CAD build for the part. Positions are in the model's coordinates, mm. A direction names the side the tool comes from. Give positions to 0.01 mm unless a question says otherwise; leave off trailing zeros. Write each loop counter-clockwise with the first axis right and the second up, starting at its lowest first coordinate (ties: lowest second). Pieces come first, ordered by that corner, then holes. Notation, with made-up numbers: (43, 55.5) - (86, 55.5) arc R11 ccw to (86, 69.5) - close; hole circle Ø5 at (23, -24). An arc over 180 degrees is marked (long way). Put each result on its own line as item: value. Start each with the question number.
1. Cut at A-A on y = -3.75. List the corners of the cut face in (x, z).
2. Cut at B-B on y = 6.5. List the corners of the cut face in (x, z), and give its area (3 significant figures).
3. Mould opens along Y. For faces 6 (the cylindrical face through (-7.166, -0.243, 4.93)), 7 (the cylindrical face through (5.31, -4.78, 4.93)), 8 (the cylindrical face through (-0.947, 8.846, 4.93)) say: +Y half, -Y half, draft (parallel to the pull), parting line (faces both ways), or undercut.
4. Drop flat-ended pins along their axis: pin 1 (1.5 mm diameter, centred on y = 3, z = 5, fed in from +X); pin 2 (5 mm diameter, centred on x = -7, z = 4.5, fed in from +Y); pin 3 (2 mm diameter, centred on x = -1.5, y = -1.5, fed in from -Z). Give the stop position or say it passes through.
5. Wall check: line 1 (X direction, y = 6.5, z = 7.25); line 2 (X direction, y = 5.75, z = 6); line 3 (X direction, y = -7.5, z = 7.5). Give the ranges that are in metal, low to high.
6. Tool access for faces 1 (the cylindrical face through (5.37, 2.46, 4.93)), 2 (the cylindrical face through (-2.14, -8.64, 4.93)), 3 (the cylindrical face through (-3.36, 6.31, 4.93)), 4 (the cylindrical face through (-3.8, -6.1, 4.9)), 5 (the cylindrical face through (8.85, 0.58, 4.93)): list every direction of +Z, -Z, +X, -X, +Y, -Y with a clear straight run to the whole face (end or side of a thin tool).
from build123d import *

# Parameters (mm, degrees)
F1_DEPTH = 10


with BuildPart() as f1:
    # F0 (on Top) → F1 (new body)
    with BuildSketch(Plane.XY):
        with BuildLine():
            ThreePointArc((1.864316, 5.3522), (1.490455, 5.713083), (1.417156, 6.227511))
            ThreePointArc((1.417156, 6.227511), (1.483836, 7.003606), (1.389552, 7.776834))
            ThreePointArc((1.389552, 7.776834), (0.955753, 8.832789), (0.188574, 9.678163))
            Line((0.188574, 9.678163), (0, 9.68))
            Line((0, 9.68), (-0.188574, 9.678163))
            ThreePointArc((-0.188574, 9.678163), (-0.955753, 8.832789), (-1.389552, 7.776834))
            ThreePointArc((-1.389552, 7.776834), (-1.483836, 7.003606), (-1.417156, 6.227511))
            ThreePointArc((-1.417156, 6.227511), (-1.490455, 5.713083), (-1.864316, 5.3522))
            ThreePointArc((-1.864316, 5.3522), (-1.900395, 5.336418), (-1.937206, 5.32243))
            ThreePointArc((-1.937206, 5.32243), (-1.974396, 5.309483), (-2.012179, 5.298382))
            ThreePointArc((-2.012179, 5.298382), (-2.530544, 5.334521), (-2.917363, 5.68148))
            ThreePointArc((-2.917363, 5.68148), (-3.365147, 6.318865), (-3.934394, 6.850587))
            ThreePointArc((-3.934394, 6.850587), (-4.945458, 7.380655), (-6.076547, 7.535116))
            Line((-6.076547, 7.535116), (-6.222184, 7.41531))
            Line((-6.222184, 7.41531), (-6.365459, 7.29269))
            ThreePointArc((-6.365459, 7.29269), (-6.409757, 6.151962), (-6.063311, 5.064213))
            ThreePointArc((-6.063311, 5.064213), (-5.638516, 4.411282), (-5.088571, 3.85962))
            ThreePointArc((-5.088571, 3.85962), (-4.814053, 3.418429), (-4.868477, 2.901664))
            ThreePointArc((-4.868477, 2.901664), (-4.88597, 2.866383), (-4.905178, 2.832006))
            ThreePointArc((-4.905178, 2.832006), (-4.925345, 2.798183), (-4.947153, 2.765393))
            ThreePointArc((-4.947153, 2.765393), (-5.367473, 2.459878), (-5.886814, 2.477022))
            ThreePointArc((-5.886814, 2.477022), (-6.63954, 2.677457), (-7.417393, 2.718875))
            ThreePointArc((-7.417393, 2.718875), (-8.532634, 2.475031), (-9.498384, 1.866304))
            Line((-9.498384, 1.866304), (-9.532939, 1.680914))
            Line((-9.532939, 1.680914), (-9.563876, 1.494886))
            ThreePointArc((-9.563876, 1.494886), (-8.864564, 0.592564), (-7.899979, -0.018009))
            ThreePointArc((-7.899979, -0.018009), (-7.154871, -0.24513), (-6.378987, -0.31423))
            ThreePointArc((-6.378987, -0.31423), (-5.885103, -0.475745), (-5.594623, -0.906593))
            ThreePointArc((-5.594623, -0.906593), (-5.585346, -0.944864), (-5.577963, -0.983545))
            ThreePointArc((-5.577963, -0.983545), (-5.571671, -1.022419), (-5.567299, -1.061555))
            ThreePointArc((-5.567299, -1.061555), (-5.692902, -1.56577), (-6.10176, -1.886463))
            ThreePointArc((-6.10176, -1.886463), (-6.807219, -2.216763), (-7.429712, -2.685029))
            ThreePointArc((-7.429712, -2.685029), (-8.127296, -3.588688), (-8.475822, -4.675772))
            Line((-8.475822, -4.675772), (-8.383126, -4.84))
            Line((-8.383126, -4.84), (-8.287248, -5.002391))
            ThreePointArc((-8.287248, -5.002391), (-7.171543, -5.244101), (-6.04016, -5.091804))
            ThreePointArc((-6.04016, -5.091804), (-5.323383, -4.786843), (-4.684605, -4.341048))
            ThreePointArc((-4.684605, -4.341048), (-4.202447, -4.147313), (-3.702983, -4.290645))
            ThreePointArc((-3.702983, -4.290645), (-3.671276, -4.313999), (-3.640757, -4.338885))
            ThreePointArc((-3.640757, -4.338885), (-3.610949, -4.364619), (-3.582444, -4.391789))
            ThreePointArc((-3.582444, -4.391789), (-3.354559, -4.858776), (-3.461625, -5.36725))
            ThreePointArc((-3.461625, -5.36725), (-3.789724, -6.073735), (-3.965586, -6.832579))
            ThreePointArc((-3.965586, -6.832579), (-3.919106, -7.973219), (-3.487328, -9.030002))
            Line((-3.487328, -9.030002), (-3.310755, -9.096225))
            Line((-3.310755, -9.096225), (-3.132925, -9.158994))
            ThreePointArc((-3.132925, -9.158994), (-2.122877, -8.626993), (-1.354082, -7.783088))
            ThreePointArc((-1.354082, -7.783088), (-1.001025, -7.088739), (-0.798243, -6.336642))
            ThreePointArc((-0.798243, -6.336642), (-0.55342, -5.878307), (-0.078676, -5.667056))
            ThreePointArc((-0.078676, -5.667056), (-0.039376, -5.664566), (0, -5.664012))
            ThreePointArc((0, -5.664012), (0.039376, -5.664566), (0.078676, -5.667056))
            ThreePointArc((0.078676, -5.667056), (0.55342, -5.878307), (0.798243, -6.336642))
            ThreePointArc((0.798243, -6.336642), (1.001025, -7.088739), (1.354082, -7.783088))
            ThreePointArc((1.354082, -7.783088), (2.122877, -8.626993), (3.132925, -9.158994))
            Line((3.132925, -9.158994), (3.310755, -9.096225))
            Line((3.310755, -9.096225), (3.487328, -9.030002))
            ThreePointArc((3.487328, -9.030002), (3.919106, -7.973219), (3.965586, -6.832579))
            ThreePointArc((3.965586, -6.832579), (3.789724, -6.073735), (3.461625, -5.36725))
            ThreePointArc((3.461625, -5.36725), (3.354559, -4.858776), (3.582444, -4.391789))
            ThreePointArc((3.582444, -4.391789), (3.610949, -4.364619), (3.640757, -4.338885))
            ThreePointArc((3.640757, -4.338885), (3.671276, -4.313999), (3.702983, -4.290645))
            ThreePointArc((3.702983, -4.290645), (4.202447, -4.147313), (4.684605, -4.341048))
            ThreePointArc((4.684605, -4.341048), (5.323383, -4.786843), (6.04016, -5.091804))
            ThreePointArc((6.04016, -5.091804), (7.171543, -5.244101), (8.287248, -5.002391))
            Line((8.287248, -5.002391), (8.383126, -4.84))
            Line((8.383126, -4.84), (8.475822, -4.675772))
            ThreePointArc((8.475822, -4.675772), (8.127296, -3.588688), (7.429712, -2.685029))
            ThreePointArc((7.429712, -2.685029), (6.807219, -2.216763), (6.10176, -1.886463))
            ThreePointArc((6.10176, -1.886463), (5.692902, -1.56577), (5.567299, -1.061555))
            ThreePointArc((5.567299, -1.061555), (5.571671, -1.022419), (5.577963, -0.983545))
            ThreePointArc((5.577963, -0.983545), (5.585346, -0.944864), (5.594623, -0.906593))
            ThreePointArc((5.594623, -0.906593), (5.885103, -0.475745), (6.378987, -0.31423))
            ThreePointArc((6.378987, -0.31423), (7.154871, -0.24513), (7.899979, -0.018009))
            ThreePointArc((7.899979, -0.018009), (8.864564, 0.592564), (9.563876, 1.494886))
            Line((9.563876, 1.494886), (9.532939, 1.680914))
            Line((9.532939, 1.680914), (9.498384, 1.866304))
            ThreePointArc((9.498384, 1.866304), (8.532634, 2.475031), (7.417393, 2.718875))
            ThreePointArc((7.417393, 2.718875), (6.63954, 2.677457), (5.886814, 2.477022))
            ThreePointArc((5.886814, 2.477022), (5.367473, 2.459878), (4.947153, 2.765393))
            ThreePointArc((4.947153, 2.765393), (4.925345, 2.798183), (4.905178, 2.832006))
            ThreePointArc((4.905178, 2.832006), (4.88597, 2.866383), (4.868477, 2.901664))
            ThreePointArc((4.868477, 2.901664), (4.814053, 3.418429), (5.088571, 3.85962))
            ThreePointArc((5.088571, 3.85962), (5.638516, 4.411282), (6.063311, 5.064213))
            ThreePointArc((6.063311, 5.064213), (6.409757, 6.151962), (6.365459, 7.29269))
            Line((6.365459, 7.29269), (6.222184, 7.41531))
            Line((6.222184, 7.41531), (6.076547, 7.535116))
            ThreePointArc((6.076547, 7.535116), (4.945458, 7.380655), (3.934394, 6.850587))
            ThreePointArc((3.934394, 6.850587), (3.365147, 6.318865), (2.917363, 5.68148))
            ThreePointArc((2.917363, 5.68148), (2.530544, 5.334521), (2.012179, 5.298382))
            ThreePointArc((2.012179, 5.298382), (1.974396, 5.309483), (1.937206, 5.32243))
            ThreePointArc((1.937206, 5.32243), (1.900395, 5.336418), (1.864316, 5.3522))
        make_face()
        Polygon((0, 5.1), (4.850388, 1.575987), (2.997705, -4.125987), (-2.997705, -4.125987), (-4.850388, 1.575987), align=None, mode=Mode.SUBTRACT)
    extrude(amount=F1_DEPTH)


solid = f1.part
Report:
1. outline: (-8.21, 0) - (-3.12, 0) - (-3.12, 10) - (-8.21, 10) - close; (3.12, 0) - (8.21, 0) - (8.21, 10) - (3.12, 10) - close
2. outline: (-6.44, 0) - (-3.53, 0) - (-3.53, 10) - (-6.44, 10) - close; (-1.46, 0) - (1.46, 0) - (1.46, 10) - (-1.46, 10) - close; (3.53, 0) - (6.44, 0) - (6.44, 10) - (3.53, 10) - close
2. area: 87.3 mm²
3. face 6: undercut
3. face 7: -Y half
3. face 8: +Y half
4. pin 1: stops at x = 8.98
4. pin 2: stops at y = 7.54
4. pin 3: passes through
5. line 1: x = -6.44 to -3.53, -1.46 to 1.46, 3.53 to 6.44
5. line 2: x = -6.33 to -2.96, -1.47 to 1.47, 2.96 to 6.33
5. line 3: x = -3.99 to -1.19, 1.19 to 3.99
6. face 1: +Z, -Z
6. face 2: +Z, -Z, -Y
6. face 3: +Z, -Z, +Y
6. face 4: +Z, -Z, -X
6. face 5: +Z, -Z, +X
